Input: part model. Units: mm. Frame: model coordinates. A direction names the side the tool comes from. Give positions to 0.01 mm unless a question says otherwise; leave off trailing zeros. Loops run counter-clockwise (first coordinate to the right, second up) from the corner with the lowest first, then second, coordinate; pieces in that order, holes last. Notation, with made-up numbers: (43, 61) - (95, 61) arc R26 cw to (95, 77) - close; hole circle Ø11 at (64, -26). An arc over 180 degrees is marked (long way). Answer as a JSON object with one key per item and string values.
from build123d import *

# Parameters (mm, degrees)
F1_W      = 431.8
F1_H      = 82.55
F2_DEPTH  = 18.2118
F4_DEPTH  = 18.2128
F6_DEPTH  = 18.2128
F7_W      = 18.2118
F7_H      = 18.2118
F7_W_2    = 25.4
F8_DEPTH  = 18.2118
F9_R      = 5.08
F10_DEPTH = 18.2128


# Not quite as in the source:
# - a variable given as a bare number and used for a length is read in inches; the dataset says mm whatever the document's units were
# - a feature names something its author has since deleted; it is built from what else it names


with BuildPart() as f2:
    # F1 (on Top) → F2 (new body)
    with BuildSketch(Plane.XY):
        Rectangle(F1_W, F1_H)
    extrude(amount=F2_DEPTH)

    # F3 (on face) → F4 (cut, through all)
    with BuildSketch(Plane.XY.offset(18.2118)):
        Polygon((-215.9, 0), (-215.9, -41.275), (-197.6882, -41.275), (-197.6882, -5.08), (-197.6882, 0), (-202.7682, 0), align=None)
        with BuildLine():
            Line((-197.6882, 0), (-197.6882, -5.08))
            ThreePointArc((-197.6882, -5.08), (-194.0960975516, 3.5921024484), (-202.7682, 0))
            Line((-202.7682, 0), (-197.6882, 0))
        make_face()
        with BuildLine():
            Line((197.6882, 0), (202.7682, 0))
            ThreePointArc((202.7682, 0), (194.0960975516, 3.5921024484), (197.6882, -5.08))
            Line((197.6882, -5.08), (197.6882, 0))
        make_face()
        Polygon((197.6882, -5.08), (197.6882, -41.275), (215.9, -41.275), (215.9, 0), (202.7682, 0), (197.6882, 0), align=None)
    extrude(amount=-F4_DEPTH, mode=Mode.SUBTRACT)

    # F5 (on face) → F6 (cut, through all)
    with BuildSketch(Plane.XY.offset(18.2118)):
        Polygon((-9.1059, -7.4021024484), (-9.1059, -41.275), (9.1059, -41.275), (9.1059, -7.4021024484), (9.1059, 0), (7.8359, 0), (-7.8359, 0), (-9.1059, 0), align=None)
        with BuildLine():
            ThreePointArc((-7.8359, 0), (-12.8610305123, -2.9478239095), (-9.1059, -7.4021024484))
            Line((-9.1059, -7.4021024484), (-9.1059, 0))
            Line((-9.1059, 0), (-7.8359, 0))
        make_face()
        with BuildLine():
            Line((9.1059, 0), (9.1059, -7.4021024484))
            ThreePointArc((9.1059, -7.4021024484), (12.8610305123, -2.9478239095), (7.8359, 0))
            Line((7.8359, 0), (9.1059, 0))
        make_face()
    extrude(amount=-F6_DEPTH, mode=Mode.SUBTRACT)

    # F7 (on face) → F8 (join)
    with BuildSketch(Plane(origin=(0, 41.275, 0), x_dir=(-1, 0, 0), z_dir=(0, 1, 0))):
        with Locations((0, 9.1059)):
            Rectangle(F7_W, F7_H)
        with Locations((-21.8059, 9.1059)):
            Rectangle(F7_W_2, F7_H)
        with Locations((21.8059, 9.1059)):
            Rectangle(F7_W_2, F7_H)
        with Locations((-206.7941, 9.1059)):
            Rectangle(F7_W, F7_H)
        with Locations((-184.9882, 9.1059)):
            Rectangle(F7_W_2, F7_H)
        with Locations((184.9882, 9.1059)):
            Rectangle(F7_W_2, F7_H)
        with Locations((206.7941, 9.1059)):
            Rectangle(F7_W, F7_H)
    extrude(amount=F8_DEPTH)

    # F9 (on face) → F10 (cut, through all)
    with BuildSketch(Plane(origin=(0, 0, 0), x_dir=(1, 0, 0), z_dir=(0, 0, -1))):
        with Locations((34.5059, -41.275)):
            Circle(F9_R)
        with Locations((-34.5059, -41.275)):
            Circle(F9_R)
        with Locations((172.2882, -41.275)):
            Circle(F9_R)
        with Locations((-172.2882, -41.275)):
            Circle(F9_R)
    extrude(amount=-F10_DEPTH, mode=Mode.SUBTRACT)


solid = f2.part
Item 1: Cut plane B-B (x = -112). Return loops of the section in (y, z) (3 decimals).
Geometry check:
{"outline": "(-41.275, 0) - (41.275, 0) - (41.275, 18.212) - (-41.275, 18.212) - close"}
Item 2: Mould query, pull axis X, two halves, no side actions, for faces 5 (the face through (215.9, 29, 9)), 6 (the face through (172.288, 53, 9)), 7 (the face through (-197.688, -23, 9)). Classes: released by +X, released by -X, zero draft, split by the parting line, or undercut.
Geometry check:
{"face 5": "released by +X", "face 6": "undercut", "face 7": "released by -X"}
Item 3: Contact query for flat-ended pins moving along their axis: P1, Ø11.5, axis at x = -34.51, y = 41.28, coming from the +Z side; P2, Ø2, axis at x = 45, z = 7, coming from the +Y side (3 decimals); P3, Ø9, axis at y = -26, z = 10.5, coming from the +X side; P4, Ø9, axis at y = -21.5, z = 11.5, coming from the -X side. Output: stop coordinate, or through.
Geometry check:
{"P1": "stops at z = 18.21", "P2": "stops at y = 41.275", "P3": "stops at x = 197.69", "P4": "stops at x = -197.69"}
Item 4: Material intervals for line 1 (X direction, y = 51.5, z = 6.75); line 2 (X direction, y = 37, z = 12.5); line 3 (X direction, y = -14, z = 14.25), sorted ascending. Write a range as [from, to].
Geometry check:
{"line 1": "x = [-215.9, -172.29], [-34.51, 34.51], [172.29, 215.9]", "line 2": "x = [-215.9, -175.03], [-169.54, -37.25], [-31.76, 31.76], [37.25, 169.54], [175.03, 215.9]", "line 3": "x = [-197.69, -9.11], [9.11, 197.69]"}
Item 5: Cut plane A-A (z = 7.5). Return loops of the section in (x, y) (3 decimals), then the cut area to 3 significant figures.
Geometry check:
{"outline": "(-215.9, 0) - (-202.768, 0) arc R5.08 cw (long way) to (-197.688, -5.08) - (-197.688, -41.275) - (-9.106, -41.275) - (-9.106, -7.402) arc R3.81 cw (long way) to (-7.836, 0) - (7.836, 0) arc R3.81 cw (long way) to (9.106, -7.402) - (9.106, -41.275) - (197.688, -41.275) - (197.688, -5.08) arc R5.08 cw (long way) to (202.768, 0) - (215.9, 0) - (215.9, 59.487) - (172.288, 59.487) - (172.288, 46.355) arc R5.08 cw (long way) to (167.208, 41.275) - (39.586, 41.275) arc R5.08 cw (long way) to (34.506, 46.355) - (34.506, 59.487) - (-34.506, 59.487) - (-34.506, 46.355) arc R5.08 cw (long way) to (-39.586, 41.275) - (-167.208, 41.275) arc R5.08 cw (long way) to (-172.288, 46.355) - (-172.288, 59.487) - (-215.9, 59.487) - close", "area": "35,800 mm2"}
Item 6: Access query for faces 1 (the face through (197.688, -23, 9)), 2 (the face through (0, 0, 9)), 3 (the face through (103, 41.275, 9)), 4 (the face through (-209, 0, 9)). Directions: +Z, -Z, +X, -X, +Y, -Y. A direction counts if a zero-diameter tool reaches every point of the face in a straight line with its end or side. Return the directions, or none.
Geometry check:
{"face 1": "+Z, -Z, +X, -Y", "face 2": "+Z, -Z, -Y", "face 3": "+Z, -Z, +Y", "face 4": "+Z, -Z, -X, -Y"}
